from build123d import *

# Parameters (mm, degrees)
F0_W     = 42
F0_H     = 17.8
F1_DEPTH = 31.2
F1_TAPER = 2
F2_R     = 11
F3_DEPTH = 25
F5_DEPTH = 3
F6_R     = 2.75
F7_DEPTH = 39.0067140634
F8_R     = 5
F8_R_2   = 2.75
F9_DEPTH = 25
F10_SIZE = 2.24999


# Not quite as in the source:
# - a fillet or chamfer is up to 0.001 mm smaller than in the source, because OpenCascade refuses the exact size


with BuildPart() as f1:
    # F0 (on Top) → F1 (new body)
    with BuildSketch(Plane.XY):
        Rectangle(F0_W, F0_H)
    extrude(amount=F1_DEPTH, taper=F1_TAPER)

    # F2 (on Right) → F3 (cut, symmetric)
    with BuildSketch(Plane.YZ):
        with Locations((0, 39.2)):
            Circle(F2_R)
    extrude(amount=F3_DEPTH, both=True, mode=Mode.SUBTRACT)

    # F4 (on face) → F5 (join)
    with BuildSketch(Plane(origin=(-20.9744225277, 0, 0.7324429743), x_dir=(0, -1, 0), z_dir=(-0.999390827, 0, 0.0348994967))):
        with BuildLine():
            Line((0, 38.2966003432), (-7.8104719919, 30.4861283514))
            Line((-7.8104719919, 30.4861283514), (-7.5498344353, 30.4861283514))
            add(Edge.make_bspline(
                [(7.5498344353, 30.4861283514), (0, 23.3567853482), (-7.5498344353, 30.4861283514)],
                knots=[2.3851362689, 2.3851362689, 2.3851362689, 3.8980490383, 3.8980490383, 3.8980490383], degree=2, weights=[1, 0.7272727273, 1]))
            Line((7.5498344353, 30.4861283514), (7.8104719919, 30.4861283514))
            Line((7.8104719919, 30.4861283514), (0, 38.2966003432))
        make_face()
    extrude(amount=-F5_DEPTH)

    # F6 (on face) → F7 (cut, through all)
    with BuildSketch(Plane(origin=(0, 0, 0), x_dir=(1, 0, 0), z_dir=(0, 0, -1))):
        with Locations((-2.25, 0)):
            Circle(F6_R)
    extrude(amount=-F7_DEPTH, mode=Mode.SUBTRACT)

    # F8 (on face) → F9 (cut)
    with BuildSketch(Plane(origin=(0, 0, 0), x_dir=(1, 0, 0), z_dir=(0, 0, -1))):
        with Locations((-2.25, 0)):
            Circle(F8_R)
        with Locations((-2.25, 0)):
            Circle(F8_R_2, mode=Mode.SUBTRACT)
    extrude(amount=-F9_DEPTH, mode=Mode.SUBTRACT)

    # F10 (size 2.25 in the source; OpenCascade refuses exactly that, so slightly less here)
    f10_edges = [f1.edges().sort_by_distance(p)[0] for p in [
        (-7.25, 0, 25),
    ]]
    chamfer(f10_edges, length=F10_SIZE)


solid = f1.part
Check sheet for the modelled part. Datum: model origin and axes. Units: mm. Round coordinates to 2 decimals unless told otherwise and drop trailing zeros. Loops run counter-clockwise (first coordinate to the right, second up) from the corner with the lowest first, then second, coordinate; pieces in that order, holes last. Notation, with made-up numbers: (68, 28) -> (116, 28) arc R19 cw to (116, 37) -> close; hole circle Ø10 at (66.5, -4). An arc over 180 degrees is marked (long way). Put each result on its own line as item: value. Start each with the question number.
1. Section check B-B (z = 19.5). Enter the section's corners in (x, y).
2. Scan lines: probe 1 along X at (y, z) = (0, 17.75); probe 2 along Y at (x, z) = (-2, 17); probe 3 along X at (y, z) = (-2.5, 23). Record each from-to range of solid material in increasing order.
3. Draft check along X on faces 1 (the face through (4, 0, 0)), 2 (the face through (-3.33, 4.88, 11.22)). Enter one of: +X half, -X half, draft (parallel to the pull), parting line (faces both ways), or undercut.
4. Section check C-C (x = 16.5). Enter the section's corners in (y, z), plus the area to 3 significant figures.
5. Section check D-D (y = 7). Enter the section's corners in (x, z), plus the area to 3 significant figures.
6. Gauge pin test, flat ends, axial feed: pin 1 (1 mm diameter, centred on x = 12, z = 29, fed in from +Y); pin 2 (6.5 mm diameter, centred on x = -2.25, y = 0, fed in from -Z); pin 3 (9 mm diameter, centred on x = -2.25, y = 0, fed in from +Z). Record the tip position at first contact, or that the pin passes through.
Findings:
1. outline: (-20.32, -8.22) -> (20.32, -8.22) -> (20.32, 8.22) -> (-20.32, 8.22) -> close; hole circle Ø10 at (-2.25, 0)
2. probe 1: x = -20.38 to -7.25, 2.75 to 20.38
2. probe 2: y = -8.31 to -4.99, 4.99 to 8.31
2. probe 3: x = -20.2 to -6.29, 1.79 to 20.2
3. face 1: draft
3. face 2: undercut
4. outline: (-8.9, 0) -> (8.9, 0) -> (7.81, 31.2) -> (7.55, 31.2) arc R11 cw to (-7.55, 31.2) -> (-7.81, 31.2) -> close
4. area: 490 mm^2
5. outline: (-21, 0) -> (21, 0) -> (19.93, 30.71) -> (-16.93, 30.71) -> (-16.88, 31.91) -> (-19.88, 32.01) -> close
5. area: 1,260 mm^2
6. pin 1: stops at y = 7.9
6. pin 2: stops at z = 24.5
6. pin 3: stops at z = 29.16
